Verification items for the finished model (mm, model axes). Give positions to 0.01 mm unless a question says otherwise; leave off trailing zeros. Order: outer loops, then holes, each group sorted by start corner. A loop starts at its lowest first (then second) coordinate and runs counter-clockwise, first axis right, second up. Notation, with made-up numbers: (46, 35.25) - (51, 35.25) arc R20 cw to (51, 47.25) - close; hole circle Ø9 at (33.5, 41). An arc over 180 degrees is marked (long way). Answer as a JSON object with one key per item and string values.
Autodesk Inventor part; units mm, degrees
ref_plane "YZ Plane" through (0, 0, 0) normal (1, 0, 0) x (0, 1, 0)
ref_plane "XZ Plane" through (0, 0, 0) normal (0, 1, 0) x (-1, 0, 0)
ref_plane "XY Plane" through (0, 0, 0) normal (0, 0, 1) x (1, 0, 0)
sketch "Boceto1" plane through (0, 0, 0) normal (0, 1, 0) x (-1, 0, 0)
  line L0 (52.5, 42.5) -> (-52.5, 42.5)
  line L1 (-52.5, 42.5) -> (-52.5, -42.5)
  line L2 (-52.5, -42.5) -> (52.5, -42.5)
  line L3 (52.5, -42.5) -> (52.5, 42.5)
  line L4 (40, 30) -> (-40, 30)
  line L5 (-40, 30) -> (-40, -30)
  line L6 (-40, -30) -> (40, -30)
  line L7 (40, -30) -> (40, 30)
  line L8 (0, -30) -> (0, -42.5)
  line L9 (52.5, 0) -> (40, 0)
  line L10 (40, 0) -> (0, 0) construction
  line L11 (0, -30) -> (0, 0) construction
  circle A0 centre (40, 30) radius 4.5
  circle A1 centre (40, -30) radius 4.5
  circle A2 centre (-40, -30) radius 4.5
  circle A3 centre (-40, 30) radius 4.5
  dimension "d0" = 105
  dimension "d1" = 85
  dimension "d4" = 80
  dimension "d5" = 60
  dimension "d6" = 9
  dimension "d7" = 9
  dimension "d8" = 9
  dimension "d9" = 9
extrude "Extrusión1" add sketch "Boceto1" along normal blind 3 contours L3 L9 L7 A0 L4 A3 L5 A2 L6 L8 L2 L1 L0 | L3 L2 L8 L6 A1 L7 L9 | L7 A1 L6 A2 L5 A3 L4 A0
properties part number "Placa_Rueda_105x85_80x60_3"
(1) Section check C-C (y = 2.05). Record the cut outline in (x, z), then the cut area to 3 significant figures.
Computed values:
{"outline": "(-52.5, -42.5) - (52.5, -42.5) - (52.5, 42.5) - (-52.5, 42.5) - close; hole circle Ø9 at (-40, -30); hole circle Ø9 at (-40, 30); hole circle Ø9 at (40, -30); hole circle Ø9 at (40, 30)", "area": "8,670 mm²"}
(2) Section check A-A (x = 40). Record the cut outline in (y, z).
Computed values:
{"outline": "(0, -42.5) - (3, -42.5) - (3, -34.5) - (0, -34.5) - close; (0, -25.5) - (3, -25.5) - (3, 25.5) - (0, 25.5) - close; (0, 34.5) - (3, 34.5) - (3, 42.5) - (0, 42.5) - close"}
(3) Material ranges on line 1 along X through (y, z) = (2.2, 30); line 2 along Z through (x, y) = (-40, 1.7); line 3 along X through (y, z) = (1.25, -27.5), recorded low to high. Write a range as [from, to].
Computed values:
{"line 1": "x = [-52.5, -44.5], [-35.5, 35.5], [44.5, 52.5]", "line 2": "z = [-42.5, -34.5], [-25.5, 25.5], [34.5, 42.5]", "line 3": "x = [-52.5, -43.74], [-36.26, 36.26], [43.74, 52.5]"}
(4) Section check B-B (z = -30). Record the cut outline in (x, y).
Computed values:
{"outline": "(-52.5, 0) - (-44.5, 0) - (-44.5, 3) - (-52.5, 3) - close; (-35.5, 0) - (35.5, 0) - (35.5, 3) - (-35.5, 3) - close; (44.5, 0) - (52.5, 0) - (52.5, 3) - (44.5, 3) - close"}
(5) Release check for a two-part mould opening along Z. For faces 1 (the cylindrical face through (37.92, 1.48, 33.99)), 2 (the flat face through (1, 1, -42.5)), 3 (the cylindrical face through (-42.08, 1.48, -26.01)), 4 (the flat face through (1, 0, 1)) record: pulls with the +Z half, pulls with the -Z half, needs draft (parallel to the pull), parting line crosses it, or undercut.
Computed values:
{"face 1": "undercut", "face 2": "pulls with the -Z half", "face 3": "undercut", "face 4": "needs draft"}
(6) Gauge pin test, flat end, axial feed: pin 1 Ø7 at (x, z) = (40, -30) entering from -Y. Record the tip position at first contact, or that the pin passes through.
Computed values:
{"pin 1": "passes through"}
